Part print with two shaded views. Sizes in mm from the minimum x, y, z corner. A direction names the side the tool comes from. Round coordinates to 2 decimals unless told otherwise and drop trailing zeros. Write each loop counter-clockwise with the first axis right and the second up, starting at its lowest first coordinate (ties: lowest second). Pieces come first, ordered by that corner, then holes. Notation, with made-up numbers: M -32.75,-36 L -11.75,-36 A28 ccw -11.75,1 Z; hole C 56.5,76.25 d7. An arc over 180 degrees is marked long. One line per question, with ' | ' between items. Start each with the question number.
1) Mould opens along Y. For the marked faces 1, 2, 3 and 4 say: pulls with the +Y half, pulls with the -Y half, needs draft (parallel to the pull), parting line crosses it, or undercut.
2) Drop flat-ended pins along their axis: pin 1 Ø2.5 at (x, y) = (64, 10.5) entering from +Z; pin 2 Ø1.5 at (x, y) = (8.5, 11) entering from +Z; pin 3 Ø1 at (y, z) = (48, 11) entering from -X. Give the stop position or say it passes through.
3) Wall check: probe 1 along Y at (x, z) = (33.92, 4.6); probe 2 along Y at (x, z) = (64.4, 3.35); probe 3 along X at (y, z) = (12, 3). Give the ranges that are in metal, low to high. Write a range as [from, to].
4) Saw through at B-B (y = 61.5). List the corners of the cut face in (x, z), plus the area to 3 significant figures.
5) Saw through at D-D (z = 18.75). List the corners of the cut face in (x, y), plus the area to 3 significant figures.
6) Saw through at A-A (z = 5). List the corners of the cut face in (x, y), plus the area to 3 significant figures.
7) Saw through at C-C (x = 33.92). List the corners of the cut face in (y, z).
8) Tool access for the marked faces 5 and 6: list every direction of +Z, -Z, +X, -X, +Y, -Y with a clear straight run to the whole face (end or side of a thin tool).
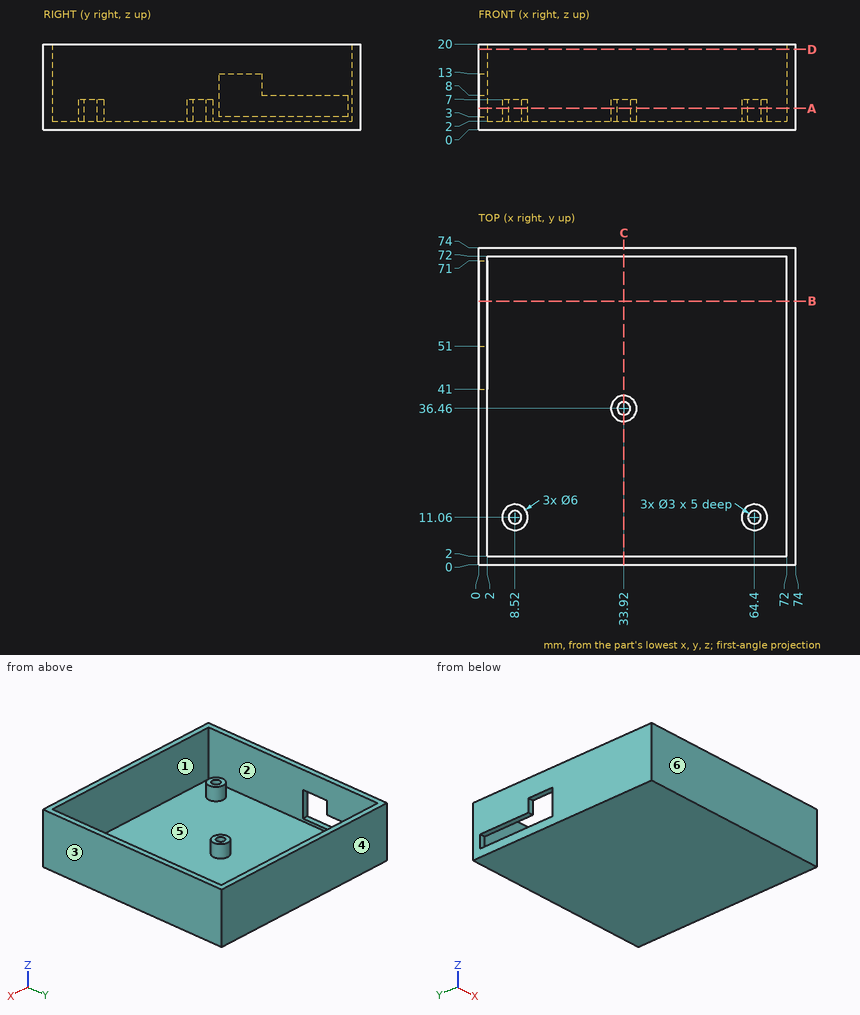
Answer key:
1) face 1: undercut | face 2: undercut | face 3: needs draft | face 4: pulls with the +Y half
2) pin 1: stops at z = 7 | pin 2: stops at z = 2 | pin 3: stops at x = 72
3) probe 1: y = [0, 2], [33.46, 34.96], [37.96, 39.46], [72, 74] | probe 2: y = [0, 2], [8.06, 9.56], [12.56, 14.06], [72, 74] | probe 3: x = [0, 2], [5.67, 7.35], [9.69, 11.37], [61.55, 63.23], [65.57, 67.25], [72, 74]
4) outline: M 0,0 L 74,0 L 74,20 L 72,20 L 72,2 L 2,2 L 2,3 L 0,3 Z; M 0,8 L 2,8 L 2,20 L 0,20 Z | area: 210 mm2
5) outline: M 0,0 L 74,0 L 74,74 L 0,74 Z; hole M 2,2 L 72,2 L 72,72 L 2,72 Z | area: 576 mm2
6) outline: M 0,0 L 74,0 L 74,74 L 0,74 L 0,71 L 2,71 L 2,72 L 72,72 L 72,2 L 2,2 L 2,41 L 0,41 Z; C 8.52,11.06 d6; C 33.92,36.46 d6; C 64.4,11.06 d6; hole C 8.52,11.06 d3; hole C 33.92,36.46 d3; hole C 64.4,11.06 d3 | area: 580 mm2
7) outline: M 0,0 L 74,0 L 74,20 L 72,20 L 72,2 L 39.46,2 L 39.46,7 L 37.96,7 L 37.96,2 L 34.96,2 L 34.96,7 L 33.46,7 L 33.46,2 L 2,2 L 2,20 L 0,20 Z
8) face 5: +Z | face 6: +Z, -Z, +X, -X, -Y
